For this review, take the finished solid that the model builds, in its own axes (mm). Give positions to 0.01 mm unless a question says otherwise; leave off trailing zeros. Write each loop counter-clockwise with the first axis right and the second up, starting at its lowest first coordinate (ties: lowest second). Pieces come first, ordered by that corner, then holes. Notation, with made-up numbers: (8.25, 76) -> (67.25, 76) arc R9 ccw to (67.25, 91) -> close; hole circle Ø8 at (-26.5, 36.5). An arc over 180 degrees is marked (long way). Return JSON: item names as keys, results as strings.
from build123d import *

# Parameters (mm, degrees)
F0_R     = 12
F0_R_2   = 7
F1_DEPTH = 15
F2_SIZE  = 1
F3_SIZE  = 0.1


with BuildPart() as f1:
    # F0 (on Top) → F1 (new body)
    with BuildSketch(Plane.XY):
        Circle(F0_R)
        Circle(F0_R_2, mode=Mode.SUBTRACT)
    extrude(amount=F1_DEPTH)

    # F2
    f2_edges = [f1.edges().sort_by_distance(p)[0] for p in [
        (-12, 0, 0),
    ]]
    chamfer(f2_edges, length=F2_SIZE)

    # F3
    f3_edges = [f1.edges().sort_by_distance(p)[0] for p in [
        (-7, 0, 0),
    ]]
    chamfer(f3_edges, length=F3_SIZE)


solid = f1.part
1. Add section A-A, the plane y = 0. State the section outline as (x, z) points, plus the area to 3 significant figures.
Results found:
{"outline": "(-12, 1) -> (-11, 0) -> (-7.1, 0) -> (-7, 0.1) -> (-7, 15) -> (-12, 15) -> close; (7, 0.1) -> (7.1, 0) -> (11, 0) -> (12, 1) -> (12, 15) -> (7, 15) -> close", "area": "149 mm²"}
2. Add section C-C, the plane z = 12. State the section outline as (x, y) points.
Results found:
{"outline": "circle Ø24 at (0, 0); hole circle Ø14 at (0, 0)"}
3. For pin 1 (1 mm diameter, centred on y = -4.5, z = 7, fed in from -X); pin 2 (3 mm diameter, centred on x = 4.5, z = 10.5, fed in from -Y); pin 3 (4 mm diameter, centred on x = -5, z = 8, fed in from +Y), all flat-tipped, find the tip position at first contact; note any pin that passes through.
Results found:
{"pin 1": "stops at x = -11.31", "pin 2": "stops at y = -11.62", "pin 3": "stops at y = 11.62"}
4. To check wall thickness, follow probe 1 along Y at (x, z) = (0, 11.25); probe 2 along X at (y, z) = (2.5, 8.25); probe 3 along X at (y, z) = (4.25, 7.5). State the ranges of each line that lie inside material, in increasing order.
Results found:
{"probe 1": "y = -12 to -7, 7 to 12", "probe 2": "x = -11.74 to -6.54, 6.54 to 11.74", "probe 3": "x = -11.22 to -5.56, 5.56 to 11.22"}
5. The part is to be moulded in two halves that separate along X. For faces 1 (the cylindrical face through (6.466, -2.681, 7.446)), 2 (the flat face through (5.2, -5.2, 15)), 3 (the cylindrical face through (-11.99, 0.53, 7.9)), say which applies: +X half, -X half, draft (parallel to the pull), parting line (faces both ways), or undercut.
Results found:
{"face 1": "undercut", "face 2": "draft", "face 3": "parting line"}
